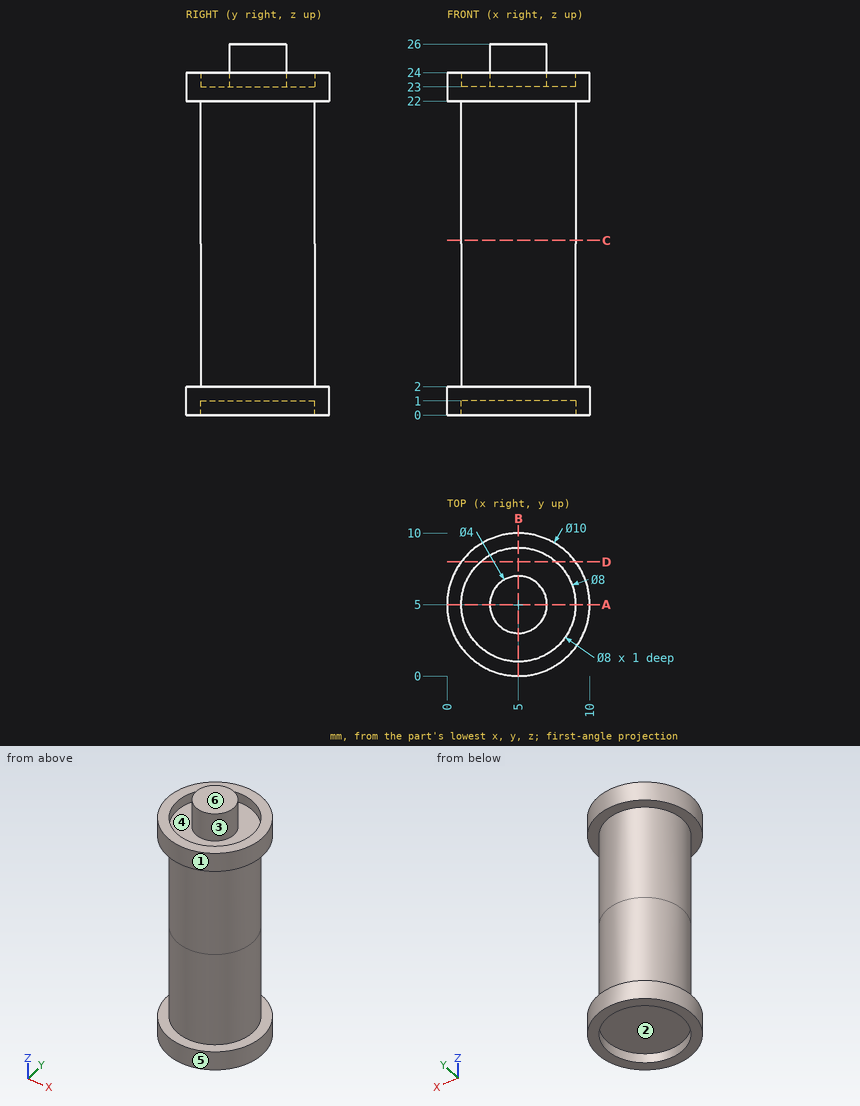
Input: dimensioned drawing with shaded views. Units: mm. Origin: part minimum x, y, z. A direction names the side the tool comes from. Give positions to 0.01 mm unless a question says otherwise; leave off trailing zeros. Write each loop counter-clockwise with the first axis right and the second up, starting at its lowest first coordinate (ties: lowest second). Pieces come first, ordered by that corner, then holes. Notation, with made-up numbers: M -22,-35.5 L -5,-35.5 A15 ccw -5,-6.5 Z; hole C 21.25,-2.75 d1. An arc over 180 degrees is marked long. Return JSON: item names as keys, results as strings. Group by question number.
1) Pin query (flat end, axial travel): P1, Ø1.5, axis at x = 5, y = 4, coming from the -Z side; P2, Ø1, axis at x = 4.5, y = 1.5, coming from the +Z side; P3, Ø3, axis at x = 3, z = 13, coming from the +Y side. Return the tip coordinate at first contact, or that it passes through.
2) Pull-direction query (X, two-part tool) for the marked faces 4, 5 and 6; classes: pulls with the +X half, pulls with the -X half, needs draft (parallel to the pull), parting line crosses it, or undercut.
3) Cut plane D-D, the plane y = 8. Output: boundary loops of the cut face in (x, z).
4) Set-up query: the marked faces 1, 2 and 3. Return all of +Z, -Z, +X, -X, +Y, -Y with unobstructed straight access to the full face (end or side cutting, diameter ignored); none if empty.
5) Material intervals for line 1 along Y through (x, z) = (5, 23.8); line 2 along Z through (x, y) = (3.5, 0.5); line 3 along Y through (x, z) = (5, 21.75), sorted ascending. Write a range as [from, to].
6) Cut plane A-A, the plane y = 5. Output: boundary loops of the cut face in (x, z), plus the area to 3 significant figures.
7) Cut plane C-C, the plane z = 12.25. Output: boundary loops of the cut face in (x, y).
Recorded:
{
 "1": {"P1": "stops at z = 1", "P2": "stops at z = 24", "P3": "stops at y = 8.97"},
 "2": {"face 4": "undercut", "face 5": "parting line crosses it", "face 6": "needs draft"},
 "3": {"outline": "M 1,0 L 2.35,0 L 2.35,1 L 7.65,1 L 7.65,0 L 9,0 L 9,2 L 7.65,2 L 7.65,22 L 9,22 L 9,24 L 7.65,24 L 7.65,23 L 2.35,23 L 2.35,24 L 1,24 L 1,22 L 2.35,22 L 2.35,2 L 1,2 Z"},
 "4": {"face 1": "+Z, -Z", "face 2": "-Z", "face 3": "+Z"},
 "5": {"line 1": "y = [0, 1], [3, 7], [9, 10]", "line 2": "z = [0, 2], [22, 24]", "line 3": "y = [1, 9]"},
 "6": {"outline": "M 0,0 L 1,0 L 1,1 L 9,1 L 9,0 L 10,0 L 10,2 L 9,2 L 9,22 L 10,22 L 10,24 L 9,24 L 9,23 L 7,23 L 7,26 L 3,26 L 3,23 L 1,23 L 1,24 L 0,24 L 0,22 L 1,22 L 1,2 L 0,2 Z", "area": "196 mm²"},
 "7": {"outline": "C 5,5 d8"}
}
